Input: dimensioned drawing with shaded views. Units: mm. Origin: part minimum x, y, z. Round coordinates to 2 decimals unless told otherwise and drop trailing zeros. Order: outer loops, then holes, each group sorted by start corner. A loop starts at its lowest first (then second) coordinate and runs counter-clockwise, first axis right, second up. Notation, with made-up numbers: (69.5, 24) - (107.5, 24) arc R7 ccw to (107.5, 35) - close; hole circle Ø3 at (2.5, -20). An arc over 180 degrees is marked (long way). One line per item, written item: value. Start each with the question number.
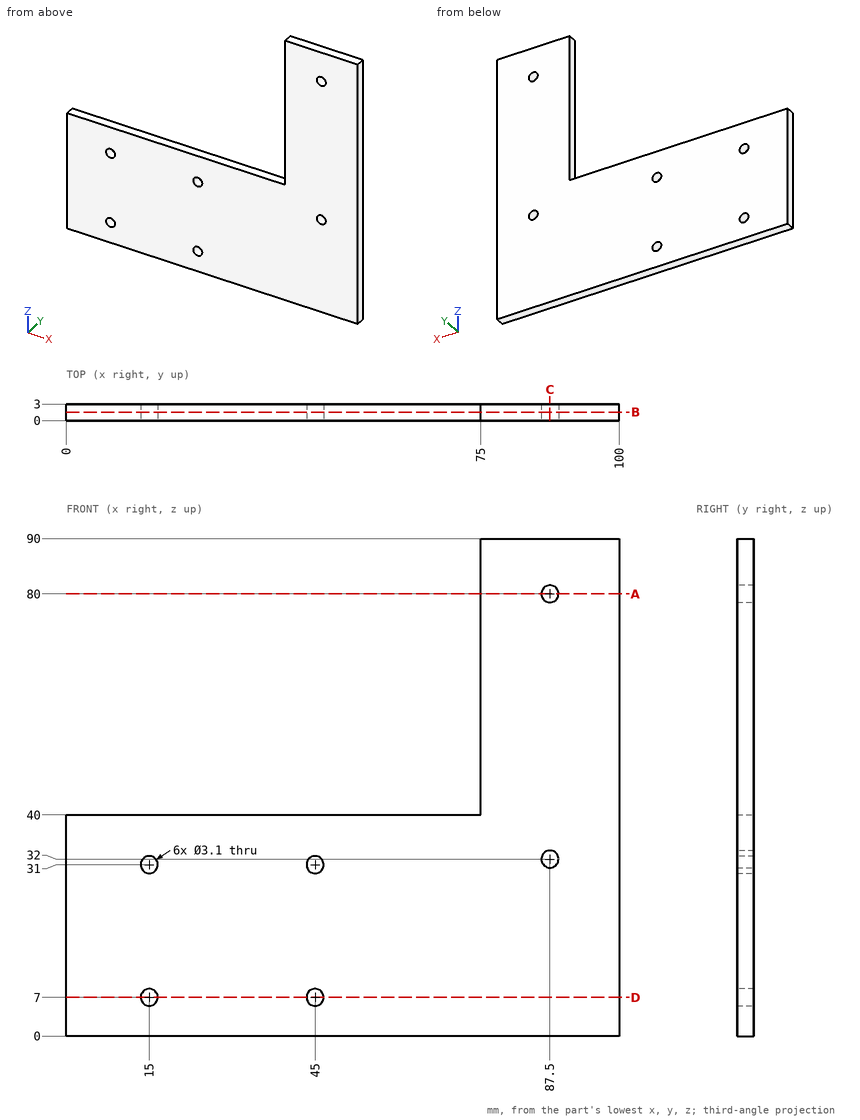
1. Section C-C (x = 87.5). Return the cut outline in (y, z).
2. Section A-A (z = 80). Return the cut outline in (x, y).
3. Pin query (flat end, axial travel): pin 1 (0.9 mm diameter, centred on y = 2, z = 59.5, fed in from -X). Return the tip coordinate at first contact, or that it passes through.
4. Section B-B (y = 1.55). Return the cut outline in (x, z).
5. Section D-D (z = 7). Return the cut outline in (x, y), then the cut area to 3 significant figures.
6. Line query: line 1 (Z direction, x = 87.5, y = 2.1); line 2 (X direction, y = 1.75, z = 7); line 3 (X direction, y = 2.05, z = 32). Output: solid intervals per line, ascending. Write a range as from..to.
Solved:
1. outline: (0, 0) - (3, 0) - (3, 30.45) - (0, 30.45) - close; (0, 33.55) - (3, 33.55) - (3, 78.45) - (0, 78.45) - close; (0, 81.55) - (3, 81.55) - (3, 90) - (0, 90) - close
2. outline: (75, 0) - (85.95, 0) - (85.95, 3) - (75, 3) - close; (89.05, 0) - (100, 0) - (100, 3) - (89.05, 3) - close
3. pin 1: stops at x = 75
4. outline: (0, 0) - (100, 0) - (100, 90) - (75, 90) - (75, 40) - (0, 40) - close; hole circle Ø3.1 at (15, 7); hole circle Ø3.1 at (15, 31); hole circle Ø3.1 at (45, 7); hole circle Ø3.1 at (45, 31); hole circle Ø3.1 at (87.5, 32); hole circle Ø3.1 at (87.5, 80)
5. outline: (0, 0) - (13.45, 0) - (13.45, 3) - (0, 3) - close; (16.55, 0) - (43.45, 0) - (43.45, 3) - (16.55, 3) - close; (46.55, 0) - (100, 0) - (100, 3) - (46.55, 3) - close
5. area: 281 mm²
6. line 1: z = 0..30.45, 33.55..78.45, 81.55..90
6. line 2: x = 0..13.45, 16.55..43.45, 46.55..100
6. line 3: x = 0..13.82, 16.18..43.82, 46.18..85.95, 89.05..100
